Part print with two shaded views. Sizes in mm from the minimum x, y, z corner. Round coordinates to 2 decimals unless told otherwise and drop trailing zeros. Write each loop counter-clockwise with the first axis right and the second up, starting at its lowest first coordinate (ties: lowest second). Pieces come first, ordered by that corner, then holes. Notation, with made-up numbers: (21, 30) -> (50, 30) arc R32 cw to (50, 58) -> close; hole circle Ø4 at (-30, 21). An arc over 180 degrees is marked (long way). Return JSON: item names as keys, results as strings. Group by question number.
(1) Saw through at B-B (z = 2.5). List the corners of the cut face in (x, y) (3 decimals).
(2) Drill centre lines: L1, parallel to Z at x = 4, y = 42; L2, parallel to Y at x = 2.5, z = 3.75; L3, parallel to Y at x = 1, z = 3.25. Where is each one in solid material? Low to high. Write a range as from..to.
(3) Drop flat-ended pins along their axis: pin 1 Ø2 at (x, z) = (3, 12.5) entering from -Y; pin 2 Ø1 at (x, z) = (13, 9) entering from +Y; pin 3 Ø1 at (y, z) = (50.5, 21) entering from -X. Give the stop position or say it passes through.
(4) Saw through at D-D (x = 11.25). List the corners of the cut face in (y, z).
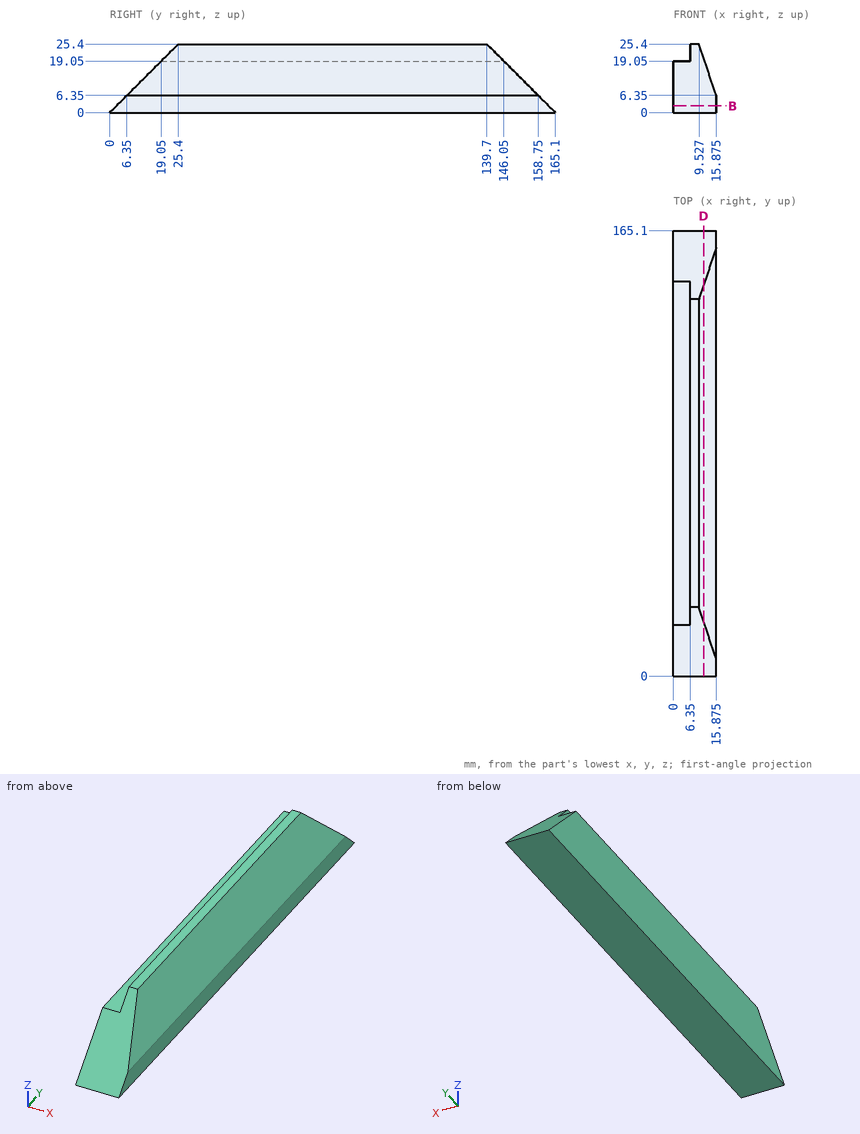
Computed values:
{
 "1": {"outline": "(0, 2.5) -> (15.875, 2.5) -> (15.875, 162.6) -> (0, 162.6) -> close"},
 "2": {"L1": "0..19.05", "L2": "3.75..161.35", "L3": "3.25..161.85"},
 "3": {"pin 1": "y = 11.5", "pin 2": "y = 156.6", "pin 3": "x = 6.35"},
 "4": {"outline": "(0, 0) -> (165.1, 0) -> (144.87, 20.23) -> (20.23, 20.23) -> close"}
}
